Source: CAD feature listing. Evaluate the final solid. Frame: model axes, mm. A direction names the side the tool comes from. Coordinates: 2 decimals unless noted, no trailing zeros. Loops run counter-clockwise (first coordinate to the right, second up) from the corner with the lowest first, then second, coordinate; pieces in that order, holes last. Notation, with made-up numbers: (26, 85) -> (66, 85) arc R15 ccw to (66, 99) -> close; hole circle Ø5 at (-30, -26). An arc over 180 degrees is marked (long way). Answer as CSV lines item,"result".
Autodesk Inventor part; units mm, degrees
ref_plane "YZ Plane" through (0, 0, 0) normal (1, 0, 0) x (0, 1, 0)
ref_plane "XZ Plane" through (0, 0, 0) normal (0, 1, 0) x (-1, 0, 0)
ref_plane "XY Plane" through (0, 0, 0) normal (0, 0, 1) x (1, 0, 0)
sketch "Sketch1" plane through (0, 0, 0) normal (0, 0, 1) x (1, 0, 0)
  line L0 (-3.5, 6) -> (-3.5, -50) construction
  line L1 (-3.5, -50) -> (0, -50) construction
  line L2 (0, -50) -> (0, 6) construction
  line L3 (-3.5, 6) -> (0, 6) construction
  line L4 (0, 0) -> (85, 0) construction
  line L5 (85, 0) -> (85, 5) construction
  line L6 (0, 5) -> (85, 5) construction
  line L7 (0, 0) -> (0, 5) construction
  line L8 (88.5, 6) -> (88.5, -50) construction
  line L9 (88.5, 6) -> (85, 6) construction
  line L10 (85, -50) -> (85, 6) construction
  line L11 (88.5, -50) -> (85, -50) construction
  line L12 (-4, 5) -> (42.5, 5)
  line L13 (42.5, 5) -> (42.5, -2)
  line L14 (42.5, -2) -> (10.6869, -5.951)
  line L15 (10.6869, -5.951) -> (3, -20)
  line L16 (3, -20) -> (-4, -20)
  line L17 (-4, -20) -> (-4, 5)
  line L18 (0, 2.5) -> (42.5, 2.5) construction
  line L19 (-2, 5) -> (-2, -20) construction
  point P0 (4.2678, 2.5)
  point P1 (21.25, 2.5)
  point P2 (-2, -0.9091)
  point P3 (-2, -16.8032)
  dimension "d0" = 4
  dimension "d1" = 25
  dimension "d2" = 7
  dimension "d3" = 7
  dimension "d7" = 2
extrude "Extrusion1" add sketch "Sketch1" along normal blind 4
sketch "Sketch2" plane through (0, 0, 4) normal (0, 0, 1) x (1, 0, 0)
  point P0 (0, 0)
  point P1 (42.5, 2.5)
  point P2 (42.5, 2.5)
  point P3 (21.25, 2.5)
  point P4 (4.2678, 2.5)
  point P5 (-2, -0.9091)
  point P6 (-2, -16.8032)
hole "Hole1" at (42.5, 2.5, 4) at (21.25, 2.5, 4) at (4.2678, 2.5, 4) at (-2, -0.9091, 4) at (-2, -16.8032, 4) direction (0, 0, -1) diameter 2 end through all
mirror "Mirror1" about plane through (42.5, -2, 0) normal (1, 0, 0)
fillet "Fillet1" radius 10 5 edges at (3, -20, 2) (10.6869, -5.951, 2) (42.5, -2, 2) (74.3131, -5.951, 2) (82, -20, 2)
properties part number "segment0c"
(1) Cut plane D-D (x = 63.75). Return the cut outline in (y, z).
Computed values:
outline,"(-4.64, 0) -> (1.5, 0) -> (1.5, 4) -> (-4.64, 4) -> close; (3.5, 0) -> (5, 0) -> (5, 4) -> (3.5, 4) -> close"
(2) Draft query along Y for faces 1 (the flat face through (-4, -8, 2)), 2 (the cylindrical face through (41.51, 2.63, 1.97)), 3 (the cylindrical face through (73.674, -7.01, 2.028)). Return one class per face: released by +Y, released by -Y, zero draft, split by the parting line, or undercut.
Computed values:
face 1,"zero draft"
face 2,"undercut"
face 3,"released by -Y"
(3) Cut plane B-B (y = -7.5). Return the cut outline in (x, z), then the cut area to 3 significant figures.
Computed values:
outline,"(-4, 0) -> (10.67, 0) -> (10.67, 4) -> (-4, 4) -> close; (74.33, 0) -> (89, 0) -> (89, 4) -> (74.33, 4) -> close"
area,"117 mm^2"
(4) Access query for faces 4 (the cylindrical face through (-1.024, -0.692, 1.972)), 5 (the flat face through (7.054, -12.591, 1.972)). Directions: +Z, -Z, +X, -X, +Y, -Y. A direction counts if a zero-diameter tool reaches every point of the face in a straight line with its end or side. Return the directions, or none.
Computed values:
face 4,"+Z, -Z"
face 5,"+Z, -Z, -Y"
(5) Cut plane A-A (y = 2.5). Return the cut outline in (x, z).
Computed values:
outline,"(-4, 0) -> (3.27, 0) -> (3.27, 4) -> (-4, 4) -> close; (5.27, 0) -> (20.25, 0) -> (20.25, 4) -> (5.27, 4) -> close; (22.25, 0) -> (41.5, 0) -> (41.5, 4) -> (22.25, 4) -> close; (43.5, 0) -> (62.75, 0) -> (62.75, 4) -> (43.5, 4) -> close; (64.75, 0) -> (79.73, 0) -> (79.73, 4) -> (64.75, 4) -> close; (81.73, 0) -> (89, 0) -> (89, 4) -> (81.73, 4) -> close"
(6) Cut plane C-C (z = 2.1). State how many separate pieces and enclosed holes the cut face has, then the cut area to 3 significant figures.
Computed values:
separate pieces,"1"
enclosed holes,"9"
area,"1,170 mm^2"
(7) Material intervals for L1, parallel to X at y = 2.5, z = 2.3; L2, parallel to X at y = -0.5, z = 1.8; L3, parallel to Y at x = 87, z = 1.9, sorted ascending. Write a range as [from, to].
Computed values:
L1,"[-4, 3.27], [5.27, 20.25], [22.25, 41.5], [43.5, 62.75], [64.75, 79.73], [81.73, 89]"
L2,"[-4, -2.91], [-1.09, 86.09], [87.91, 89]"
L3,"[-19.96, -17.8], [-15.8, -1.91], [0.09, 5]"
